```python
from build123d import *

# Parameters (mm, degrees)
F3_DEPTH = 25


# Not quite as in the source:
# - a fillet or chamfer that OpenCascade refuses, or shapes differently, is made with other operations: its cross-section is extruded or revolved along the edge and cut away or added


with BuildPart() as f1:
    # F0 (on Front) → F1 (revolve)
    with BuildSketch(Plane.XZ):
        Polygon((22.8, -3), (23.8, -3), (23.8, 0), (42, 0), (42, 1), (22.8, 1), align=None)
    revolve(axis=Axis((0, 0, 4.016155377), (0, 0, 1)))

    # F2 (on Top) → F3 (cut)
    with BuildSketch(Plane.XY):
        Polygon((-5, 30), (0, 30), (5, 30), (5, 35), (-5, 35), align=None)
    extrude(amount=F3_DEPTH, mode=Mode.SUBTRACT)

    # F4: fillet of radius 2 on 1 edges, made by hand

    # F4_s1 → F4_t2 (revolve, cut)
    with BuildSketch(Plane.XZ):
        with BuildLine():
            ThreePointArc((23.8, -3), (23.0679491924, -2.2679491924), (22.8, -1.2679491924))
            Line((22.8, -1.2679491924), (22.8, -3))
            Line((22.8, -3), (23.8, -3))
        make_face()
    revolve(axis=Axis((0, 0, -3), (0, 0, 1)), mode=Mode.SUBTRACT)


solid = f1.part
```
Part model, mm, in its own coordinate system. A direction names the side the tool comes from. Coordinates: 2 decimals unless noted, no trailing zeros. Loops run counter-clockwise (first coordinate to the right, second up) from the corner with the lowest first, then second, coordinate; pieces in that order, holes last. Notation, with made-up numbers: (19, 22) - (76, 22) arc R7 cw to (76, 31) - close; hole circle Ø4 at (16.5, -17.75). An arc over 180 degrees is marked (long way). Write item = value, one per line. Start each with the question number.
Item 1: Cut at D-D, the plane y = 32. Give the cut face in (x, z).
Item 2: Cut at A-A, the plane y = 0. Give the cut face in (x, z), and give its area (3 significant figures).
Item 3: 3-axis set-ups, long thin cutter, end or side, ignore diameter. For faces 1 (the flat face through (18, -18, 1)), 2 (the cylindrical face through (-17.542, 16.085, -1.479)): which of +Z, -Z, +X, -X, +Y, -Y reach the whole face in a straight line?
Item 4: Mould opens along Y. For faces 3 (the cylindrical face through (40.06, 12.62, 0.51)), 4 (the cylindrical face through (-18.093, -13.873, -0.15)), 5 (the flat face through (-18, -18, 0)) say: released by +Y, released by -Y, zero draft, split by the parting line, or undercut.
Item 5: Flat gauge pins, fed straight in: pin 1 Ø0.5 at (y, z) = (33.5, 0.5) entering from +X; pin 2 Ø8 at (x, y) = (32.5, 26) entering from -Z; pin 3 Ø1.5 at (x, z) = (9.5, -1.5) entering from -Y. Where does each tip first touch, or does it go through?
Item 6: Cut at C-C, the plane z = -0.6. Give the cut face in (x, y).
Item 7: Wall check: L1, parallel to Y at x = 0, z = 0.4; L2, parallel to Y at x = 0, z = -0.6; L3, parallel to Z at x = 30, y = -5.5. Give the ranges that are in metal, low to high. Write a range as from..to.
Item 8: Cut at B-B, the plane x = 0. Give the cut face in (y, z), and give its area (3 significant figures).
The answers:
q1.outline = (-27.2, 0) - (-5, 0) - (-5, 1) - (-27.2, 1) - close; (5, 0) - (27.2, 0) - (27.2, 1) - (5, 1) - close
q2.outline = (-42, 0) - (-23.8, 0) - (-23.8, -3) arc R2 ccw to (-22.8, -1.27) - (-22.8, 1) - (-42, 1) - close; (22.8, -1.27) arc R2 ccw to (23.8, -3) - (23.8, 0) - (42, 0) - (42, 1) - (22.8, 1) - close
q2.area = 43.4 mm2
q3.face_1 = +Z, +X, -X, +Y, -Y
q3.face_2 = -Z
q4.face_3 = split by the parting line
q4.face_4 = undercut
q4.face_5 = zero draft
q5.pin_1 = 25.66
q5.pin_2 = 0
q5.pin_3 = -22.13
q6.outline = circle Ø47.6 at (0, 0); hole circle Ø45.6 at (0, 0)
q7.L1 = -42..-22.8, 22.8..30, 35..42
q7.L2 = -23.8..-22.8, 22.8..23.8
q7.L3 = 0..1
q8.outline = (-42, 0) - (-23.8, 0) - (-23.8, -3) arc R2 ccw to (-22.8, -1.27) - (-22.8, 1) - (-42, 1) - close; (22.8, -1.27) arc R2 ccw to (23.8, -3) - (23.8, 0) - (30, 0) - (30, 1) - (22.8, 1) - close; (35, 0) - (42, 0) - (42, 1) - (35, 1) - close
q8.area = 38.4 mm2
